Build history of the part. All positions in model axes, mm. A direction names the side the tool comes from. Round coordinates to 2 decimals unless told otherwise and drop trailing zeros. Write each loop counter-clockwise with the first axis right and the second up, starting at its lowest first coordinate (ties: lowest second). Pieces come first, ordered by that corner, then holes. Notation, with made-up numbers: M 33.5,69.5 L 68.5,69.5 A9 ccw 68.5,76.5 Z; hole C 41,-5 d5. An arc over 180 degrees is marked long. Use a Markdown table: item, result.
from build123d import *

# Parameters (mm, degrees)
SKETCH_1_W          = 17.14
SKETCH_1_H          = 11
EXTRUDE_1_DEPTH     = 10
CUT_EXTRUDE_1_DEPTH = 18.159396843
CUT_EXTRUDE_2_DEPTH = 1.75
SKETCH_4_R          = 1.5
CUT_EXTRUDE_3_DEPTH = 14.105624747


with BuildPart() as part:
    # 草图1 → 凸台-拉伸1 (new body)
    with BuildSketch(Plane(origin=(0, 0, 0), x_dir=(1, 0, 0), z_dir=(0, 1, 0))):
        Rectangle(SKETCH_1_W, SKETCH_1_H)
    extrude(amount=EXTRUDE_1_DEPTH)

    # 草图2 → 切除-拉伸1 (cut, through all)
    with BuildSketch(Plane.XY.offset(5.5)):
        with BuildLine():
            Line((-6.87, 10), (-7.87, 10))
            Line((-7.87, 10), (-7.87, 2.5))
            ThreePointArc((-7.87, 2.5), (-7.37, 3), (-6.87, 2.5))
            Line((-6.87, 2.5), (-6.87, 10))
        make_face()
        with BuildLine():
            Line((-5.27, 10), (-6.27, 10))
            Line((-6.27, 10), (-6.27, 2.5))
            ThreePointArc((-6.27, 2.5), (-5.77, 3), (-5.27, 2.5))
            Line((-5.27, 2.5), (-5.27, 10))
        make_face()
        with BuildLine():
            ThreePointArc((-6.87, 2.5), (-7.37, 3), (-7.87, 2.5))
            Line((-7.87, 2.5), (-6.87, 2.5))
        make_face()
        with BuildLine():
            Line((-6.87, 2.5), (-7.87, 2.5))
            ThreePointArc((-7.87, 2.5), (-7.37, 2), (-6.87, 2.5))
        make_face()
        with BuildLine():
            ThreePointArc((-5.27, 2.5), (-5.77, 3), (-6.27, 2.5))
            Line((-6.27, 2.5), (-5.27, 2.5))
        make_face()
        with BuildLine():
            Line((-5.27, 2.5), (-6.27, 2.5))
            ThreePointArc((-6.27, 2.5), (-5.77, 2), (-5.27, 2.5))
        make_face()
        with BuildLine():
            Line((-3.67, 10), (-4.67, 10))
            Line((-4.67, 10), (-4.67, 2.5))
            ThreePointArc((-4.67, 2.5), (-4.17, 3), (-3.67, 2.5))
            Line((-3.67, 2.5), (-3.67, 10))
        make_face()
        with BuildLine():
            ThreePointArc((-3.67, 2.5), (-4.17, 3), (-4.67, 2.5))
            Line((-4.67, 2.5), (-3.67, 2.5))
        make_face()
        with BuildLine():
            Line((-3.67, 2.5), (-4.67, 2.5))
            ThreePointArc((-4.67, 2.5), (-4.17, 2), (-3.67, 2.5))
        make_face()
        with BuildLine():
            Line((-2.07, 10), (-3.07, 10))
            Line((-3.07, 10), (-3.07, 2.5))
            ThreePointArc((-3.07, 2.5), (-2.57, 3), (-2.07, 2.5))
            Line((-2.07, 2.5), (-2.07, 10))
        make_face()
        with BuildLine():
            ThreePointArc((-2.07, 2.5), (-2.57, 3), (-3.07, 2.5))
            Line((-3.07, 2.5), (-2.07, 2.5))
        make_face()
        with BuildLine():
            Line((-2.07, 2.5), (-3.07, 2.5))
            ThreePointArc((-3.07, 2.5), (-2.57, 2), (-2.07, 2.5))
        make_face()
        with BuildLine():
            Line((-0.47, 10), (-1.47, 10))
            Line((-1.47, 10), (-1.47, 2.5))
            ThreePointArc((-1.47, 2.5), (-0.97, 3), (-0.47, 2.5))
            Line((-0.47, 2.5), (-0.47, 10))
        make_face()
        with BuildLine():
            ThreePointArc((-0.47, 2.5), (-0.97, 3), (-1.47, 2.5))
            Line((-1.47, 2.5), (-0.47, 2.5))
        make_face()
        with BuildLine():
            Line((-0.47, 2.5), (-1.47, 2.5))
            ThreePointArc((-1.47, 2.5), (-0.97, 2), (-0.47, 2.5))
        make_face()
        with BuildLine():
            Line((1.13, 10), (0.13, 10))
            Line((0.13, 10), (0.13, 2.5))
            ThreePointArc((0.13, 2.5), (0.63, 3), (1.13, 2.5))
            Line((1.13, 2.5), (1.13, 10))
        make_face()
        with BuildLine():
            ThreePointArc((1.13, 2.5), (0.63, 3), (0.13, 2.5))
            Line((0.13, 2.5), (1.13, 2.5))
        make_face()
        with BuildLine():
            Line((1.13, 2.5), (0.13, 2.5))
            ThreePointArc((0.13, 2.5), (0.63, 2), (1.13, 2.5))
        make_face()
        with BuildLine():
            Line((2.73, 10), (1.73, 10))
            Line((1.73, 10), (1.73, 2.5))
            ThreePointArc((1.73, 2.5), (2.23, 3), (2.73, 2.5))
            Line((2.73, 2.5), (2.73, 10))
        make_face()
        with BuildLine():
            ThreePointArc((2.73, 2.5), (2.23, 3), (1.73, 2.5))
            Line((1.73, 2.5), (2.73, 2.5))
        make_face()
        with BuildLine():
            Line((2.73, 2.5), (1.73, 2.5))
            ThreePointArc((1.73, 2.5), (2.23, 2), (2.73, 2.5))
        make_face()
        with BuildLine():
            Line((4.33, 10), (3.33, 10))
            Line((3.33, 10), (3.33, 2.5))
            ThreePointArc((3.33, 2.5), (3.83, 3), (4.33, 2.5))
            Line((4.33, 2.5), (4.33, 10))
        make_face()
        with BuildLine():
            ThreePointArc((4.33, 2.5), (3.83, 3), (3.33, 2.5))
            Line((3.33, 2.5), (4.33, 2.5))
        make_face()
        with BuildLine():
            Line((4.33, 2.5), (3.33, 2.5))
            ThreePointArc((3.33, 2.5), (3.83, 2), (4.33, 2.5))
        make_face()
        with BuildLine():
            Line((5.93, 10), (4.93, 10))
            Line((4.93, 10), (4.93, 2.5))
            ThreePointArc((4.93, 2.5), (5.43, 3), (5.93, 2.5))
            Line((5.93, 2.5), (5.93, 10))
        make_face()
        with BuildLine():
            ThreePointArc((5.93, 2.5), (5.43, 3), (4.93, 2.5))
            Line((4.93, 2.5), (5.93, 2.5))
        make_face()
        with BuildLine():
            Line((5.93, 2.5), (4.93, 2.5))
            ThreePointArc((4.93, 2.5), (5.43, 2), (5.93, 2.5))
        make_face()
        with BuildLine():
            Line((7.53, 10), (6.53, 10))
            Line((6.53, 10), (6.53, 2.5))
            ThreePointArc((6.53, 2.5), (7.03, 3), (7.53, 2.5))
            Line((7.53, 2.5), (7.53, 10))
        make_face()
        with BuildLine():
            ThreePointArc((7.53, 2.5), (7.03, 3), (6.53, 2.5))
            Line((6.53, 2.5), (7.53, 2.5))
        make_face()
        with BuildLine():
            Line((7.53, 2.5), (6.53, 2.5))
            ThreePointArc((6.53, 2.5), (7.03, 2), (7.53, 2.5))
        make_face()
    extrude(amount=-CUT_EXTRUDE_1_DEPTH, mode=Mode.SUBTRACT)

    # 草图3 → 切除-拉伸2 (cut)
    with BuildSketch(Plane.XZ):
        with BuildLine():
            ThreePointArc((2.23, 3.65), (1.995685425, 4.215685425), (1.43, 4.45))
            Line((1.43, 4.45), (1.43, 2.85))
            ThreePointArc((1.43, 2.85), (1.995685425, 3.084314575), (2.23, 3.65))
        make_face()
        with BuildLine():
            Line((1.43, 2.85), (1.43, 4.45))
            ThreePointArc((1.43, 4.45), (0.63, 3.65), (1.43, 2.85))
        make_face()
        with BuildLine():
            ThreePointArc((2.23, -3.65), (1.995685425, -3.084314575), (1.43, -2.85))
            Line((1.43, -2.85), (1.43, -4.45))
            ThreePointArc((1.43, -4.45), (1.995685425, -4.215685425), (2.23, -3.65))
        make_face()
        with BuildLine():
            Line((1.43, -4.45), (1.43, -2.85))
            ThreePointArc((1.43, -2.85), (0.63, -3.65), (1.43, -4.45))
        make_face()
    extrude(amount=-CUT_EXTRUDE_2_DEPTH, mode=Mode.SUBTRACT)

    # 草图4 → 切除-拉伸3 (cut, through all)
    with BuildSketch(Plane.XZ.offset(-1.75)):
        with Locations(Location((1.43, 3.65, 0), (0, 0, 270))):
            Circle(SKETCH_4_R)
        with Locations(Location((1.43, -3.65, 0), (0, 0, 270))):
            Circle(SKETCH_4_R)
    extrude(amount=-CUT_EXTRUDE_3_DEPTH, mode=Mode.SUBTRACT)


solid = part.part
Q1. Cut at A-A on y = 0.5. Give the cut face in (x, z), and give its area (3 significant figures).
Response values:
| item | result |
|---|---|
| outline | M -8.57,-5.5 L 8.57,-5.5 L 8.57,5.5 L -8.57,5.5 Z; hole C 1.43,-3.65 d1.6; hole C 1.43,3.65 d1.6 |
| area | 185 mm2 |
Q2. Which spindle directions (+Z, -Z, +X, -X, +Y, -Y) get a long thin tool onto all of the face, cutting with end or side? Do faces 3 (the flat face through (6.53, 6, 0)), 4 (the flat face through (8.57, 5, 0)), 5 (the cylindrical face through (-0.034, 5.817, -3.325)). Say none if no direction does.
Response values:
| item | result |
|---|---|
| face 3 | +Z, -Z, +Y |
| face 4 | +Z, -Z, +X, +Y, -Y |
| face 5 | +Y |
Q3. Drill centre lines: L1, parallel to Y at x = -3, z = -1.75; L2, parallel to Y at x = 3.75, z = 1.25. Where is each one in solid material? Low to high.
Response values:
| item | result |
|---|---|
| L1 | y = 0 to 2.24 |
| L2 | y = 0 to 2.01 |
Q4. Two-plate mould, pull along Z, no slides. Class faces 1 (the flat face through (0.45, 1.75, 3.67)), 2 (the flat face through (0, 0, 0)): +Z half, -Z half, draft (parallel to the pull), parting line (faces both ways), or undercut.
Response values:
| item | result |
|---|---|
| face 1 | undercut |
| face 2 | draft |
Q5. Cut at C-C on x = -5.77. Give the cut face in (y, z).
Response values:
| item | result |
|---|---|
| outline | M 0,-5.5 L 2,-5.5 L 2,5.5 L 0,5.5 Z |
Q6. Cut at B-B on y = 3.5. Count the separate pieces of the cut face and the enclosed holes in it, and give its area (3 significant figures).
Response values:
| item | result |
|---|---|
| separate pieces | 13 |
| enclosed holes | 0 |
| area | 74.2 mm2 |
